Design review of the part built by this model. Coordinates are the model's own, in mm. A direction names the side the tool comes from. Round coordinates to 2 decimals unless told otherwise and drop trailing zeros. Loops run counter-clockwise (first coordinate to the right, second up) from the corner with the lowest first, then second, coordinate; pieces in that order, holes last. Notation, with made-up numbers: (75, 23.5) - (94, 23.5) arc R25 ccw to (94, 35.5) - close; hole circle Ø1 at (-7.75, 11.5). An arc over 180 degrees is marked (long way). Answer as CSV lines item,"result". Start each with the question number.
(1) Consider section D-D (x = 7.75). Give the boundary of the cut face in (y, z).
(2) Mouldability with a two-part tool opening along Y and no side actions: class faces 4 (the flat face through (0, 145.5, 0)), 5 (the flat face through (-10, 10, 0)), 6 (the flat face through (2.2, 143, -0.1)) as released by +Y, released by -Y, zero draft, split by the parting line, or undercut.
(3) Consider section A-A (z = 0). Give the boundary of the cut face in (x, y), and give its area (3 significant figures).
(4) For faces 1 (the cylindrical face through (0, 141, -2)), 2 (the flat face through (0, 10, 10)), 3 (the cylindrical face through (4.38, 79.16, -8.43)), list the 3-axis set-ups (+Z, -Z, +X, -X, +Y, -Y) from which the entire face can be reached by the end or side of a thin tool; tool diameter is ignored.
(5) Consider section B-B (x = 0). Give the boundary of the cut face in (y, z), and give its area (3 significant figures).
(6) Wall thickness on L1, parallel to Y at x = 0.75, z = 2.25; L2, parallel to Y at x = 8.75, z = 0.75; L3, parallel to Y at x = -7.75, z = -8.25: over which ranges is each line inside the solid? List them lowest first.
(7) For P1, Ø10, axis at y = 26.5, z = -2.5, coming from the +X side; P2, Ø4, axis at x = -2, y = 69.5, coming from the -Z side; P3, Ø1, axis at y = 37.5, z = -2.5, coming from the +X side; P4, Ø2, axis at x = 5, z = 3, coming from the +Y side, all flat-tipped, find the tip position at first contact; note any pin that passes through.
(8) Consider section C-C (y = 75). Give the boundary of the cut face in (x, z).
Autodesk Inventor part; units mm, degrees
ref_plane "YZ Plane" through (0, 0, 0) normal (1, 0, 0) x (0, 1, 0)
ref_plane "XZ Plane" through (0, 0, 0) normal (0, 1, 0) x (-1, 0, 0)
ref_plane "XY Plane" through (0, 0, 0) normal (0, 0, 1) x (1, 0, 0)
sketch "Sketch1" plane through (0, 0, 0) normal (0, 1, 0) x (-1, 0, 0)
  line L0 (-10, 10) -> (10, 10)
  line L1 (10, 10) -> (10, -10)
  line L2 (10, -10) -> (-10, -10)
  line L3 (-10, -10) -> (-10, 10)
  line L4 (-10, 10) -> (10, -10) construction
  line L5 (10, 10) -> (-10, -10) construction
  point P0 (0, 0)
  dimension "d0" = 20
  dimension "d1" = 20
extrude "Extrusion1" add sketch "Sketch1" along normal blind 20
sketch "Sketch2" plane through (0, 20, 0) normal (0, 1, 0) x (1, 0, 0)
  circle A0 centre (0, 0) radius 9.5
  dimension "d4" = 19
extrude "Extrusion2" add sketch "Sketch2" along normal blind 120
sketch "Sketch3" plane through (0, 140, 0) normal (0, 1, 0) x (1, 0, 0)
  circle A0 centre (0, 0) radius 2
  dimension "d7" = 4
extrude "Extrusion3" add sketch "Sketch3" along normal blind 3
sketch "Sketch4" plane through (0, 143, 0) normal (0, 1, 0) x (1, 0, 0)
  circle A0 centre (0, 0) radius 5
  dimension "d10" = 10
extrude "Extrusion4" add sketch "Sketch4" along normal blind 2.5
thread "Thread1"
properties part number "Trapezspindle" material "Steel"
Determined:
1,outline,"(0, -10) - (20, -10) - (20, -5.49) - (140, -5.49) - (140, 5.49) - (20, 5.49) - (20, 10) - (0, 10) - close"
2,face 4,"released by +Y"
2,face 5,"zero draft"
2,face 6,"undercut"
3,outline,"(-10, 0) - (10, 0) - (10, 20) - (9.5, 20) - (9.5, 140) - (2, 140) - (2, 143) - (5, 143) - (5, 145.5) - (-5, 145.5) - (-5, 143) - (-2, 143) - (-2, 140) - (-9.5, 140) - (-9.5, 20) - (-10, 20) - close"
3,area,"2,720 mm^2"
4,face 1,"none"
4,face 2,"+Z, +X, -X, +Y, -Y"
4,face 3,"+Y"
5,outline,"(0, -10) - (20, -10) - (20, -9.5) - (140, -9.5) - (140, -2) - (143, -2) - (143, -5) - (145.5, -5) - (145.5, 5) - (143, 5) - (143, 2) - (140, 2) - (140, 9.5) - (20, 9.5) - (20, 10) - (0, 10) - close"
5,area,"2,720 mm^2"
6,L1,"y = 0 to 140, 143 to 145.5"
6,L2,"y = 0 to 140"
6,L3,"y = 0 to 20"
7,P1,"stops at x = 9.5"
7,P2,"stops at z = -9.5"
7,P3,"stops at x = 9.29"
7,P4,"stops at y = 145.5"
8,outline,"circle Ø19 at (0, 0)"
